from build123d import *

# Parameters (mm, degrees)
SKETCH_1_W          = 26
SKETCH_1_H          = 57.5
SKETCH_1_R          = 1.5
SKETCH_1_R_2        = 6
EXTRUDE_1_DEPTH     = 3
SKETCH_2_W          = 26
SKETCH_2_H          = 3
EXTRUDE_2_DEPTH     = 33
SKETCH_3_W          = 34
SKETCH_3_H          = 60.5
SKETCH_3_R          = 2
SKETCH_3_R_2        = 13
EXTRUDE_3_DEPTH     = 3
FILLET_1_R          = 2
EXTRUDE_4_DEPTH     = 1
FILLET_2_R          = 4
SKETCH_5_R          = 1.5
CUT_EXTRUDE_1_DEPTH = 50.503156465


with BuildPart() as part:
    # 草图1 → 凸台-拉伸1 (new body)
    with BuildSketch(Plane.XY):
        Rectangle(SKETCH_1_W, SKETCH_1_H)
        with Locations((-5, 24.25)):
            Circle(SKETCH_1_R, mode=Mode.SUBTRACT)
        with Locations((5, 24.25)):
            Circle(SKETCH_1_R, mode=Mode.SUBTRACT)
        with Locations((5, -24.25)):
            Circle(SKETCH_1_R, mode=Mode.SUBTRACT)
        with Locations((-5, -24.25)):
            Circle(SKETCH_1_R, mode=Mode.SUBTRACT)
        with Locations((0, 10.25)):
            Circle(SKETCH_1_R_2, mode=Mode.SUBTRACT)
    extrude(amount=EXTRUDE_1_DEPTH)

    # 草图2 → 凸台-拉伸2 (add)
    with BuildSketch(Plane(origin=(0, 0, 0), x_dir=(-1, 0, 0), z_dir=(0, 0, -1))):
        with Locations((0, -30.25)):
            Rectangle(SKETCH_2_W, SKETCH_2_H)
    extrude(amount=-EXTRUDE_2_DEPTH)

    # 草图3 → 凸台-拉伸3 (add)
    with BuildSketch(Plane.XY.offset(33)):
        with Locations((0, -1.5)):
            Rectangle(SKETCH_3_W, SKETCH_3_H)
        with Locations((12.374368671, 22.624368671)):
            Circle(SKETCH_3_R, mode=Mode.SUBTRACT)
        with Locations((12.374368671, -2.124368671)):
            Circle(SKETCH_3_R, mode=Mode.SUBTRACT)
        with Locations((-12.374368671, -2.124368671)):
            Circle(SKETCH_3_R, mode=Mode.SUBTRACT)
        with Locations((-12.374368671, 22.624368671)):
            Circle(SKETCH_3_R, mode=Mode.SUBTRACT)
        with Locations((0, 10.25)):
            Circle(SKETCH_3_R_2, mode=Mode.SUBTRACT)
    extrude(amount=-EXTRUDE_3_DEPTH)

    # 圆角1
    fillet_1_edges = [part.edges().sort_by_distance(p)[0] for p in [
        (0, -28.75, 3),
        (0, -28.75, 30),
    ]]
    fillet(fillet_1_edges, radius=FILLET_1_R)

    # 草图4 → 凸台-拉伸4 (add)
    with BuildSketch(Plane.XZ.offset(31.75)):
        Polygon((13, 0), (13, 30), (17, 30), (17, 33), (-17, 33), (-17, 30), (-13, 30), (-13, 0), align=None)
    extrude(amount=EXTRUDE_4_DEPTH)

    # 圆角2
    fillet_2_edges = [part.edges().sort_by_distance(p)[0] for p in [
        (-13, 28.75, 1.5),
        (13, 28.75, 1.5),
        (-17, 28.75, 31.5),
        (17, 28.75, 31.5),
        (17, -32.75, 31.5),
        (-17, -32.75, 31.5),
    ]]
    fillet(fillet_2_edges, radius=FILLET_2_R)

    # 草图5 → 切除-拉伸1 (cut, through all)
    with BuildSketch(Plane(origin=(0, 0, 0), x_dir=(-1, 0, 0), z_dir=(0, 0, -1))):
        with Locations(Location((-5, -24.25, 0), (0, 0, 180))):
            Circle(SKETCH_5_R)
        with Locations(Location((5, -24.25, 0), (0, 0, 180))):
            Circle(SKETCH_5_R)
        with Locations((-5, -14.244897428)):
            Circle(SKETCH_5_R)
        with Locations((5, -14.244897428)):
            Circle(SKETCH_5_R)
    extrude(amount=-CUT_EXTRUDE_1_DEPTH, mode=Mode.SUBTRACT)


solid = part.part
Part model, mm, in its own coordinate system. A direction names the side the tool comes from. Give positions to 0.01 mm unless a question says otherwise; leave off trailing zeros. Loops run counter-clockwise (first coordinate to the right, second up) from the corner with the lowest first, then second, coordinate; pieces in that order, holes last.
(1) 3-axis set-ups, long thin cutter, end or side, ignore diameter. For faces 1 (the cylindrical face through (-10.316, 2.34, 31.521)), 2 (the cylindrical face through (0.18, -28.15, 3.57)), 3 (the cylindrical face through (-15.859, 27.547, 31.479)): which of +Z, -Z, +X, -X, +Y, -Y reach the whole face in a straight line?
Return value:
face 1: +Z
face 2: +X, -X, +Y
face 3: +Z, -Z, -X, +Y
(2) Pull direction X, two halves, no side cores. Call faces 4 (the flat face through (0, 28.75, 1)), 5 (the cylindrical face through (4.805, -25.737, 31.479)), 6 (the cylindrical face through (11.859, 27.547, 1.521)): pulls with the +X half, pulls with the -X half, needs draft (parallel to the pull), parting line crosses it, or undercut.
Return value:
face 4: needs draft
face 5: undercut
face 6: pulls with the +X half
(3) Band-saw the part on D-D (z = 15.5). Write the cut outline in (x, y), and give its area (3 significant figures).
Return value:
outline: (-13, -32.75) - (13, -32.75) - (13, -28.75) - (-13, -28.75) - close
area: 104 mm2
(4) Band-saw the part on B-B (y = 10.25). Write the cut outline in (x, z).
Return value:
outline: (-17, 30) - (-13, 30) - (-13, 33) - (-17, 33) - close; (-13, 0) - (-6, 0) - (-6, 3) - (-13, 3) - close; (6, 0) - (13, 0) - (13, 3) - (6, 3) - close; (13, 30) - (17, 30) - (17, 33) - (13, 33) - close
(5) Pin check, flat tips, straight feed: pin 1 (3 mm diameter, centred on x = 2, y = 0.5, fed in from +Z); pin 2 (9 mm diameter, centred on y = 2.5, z = 22.5, fed in from -X); pin 3 (7 mm diameter, centred on x = 0.5, z = 15.5, fed in from +Y). Stop position of each tip, or through.
Return value:
pin 1: stops at z = 3
pin 2: passes through
pin 3: stops at y = -28.75
(6) Band-saw the part on A-A (x = 0). Write the cut outline in (y, z), and give its area (3 significant figures).
Return value:
outline: (-32.75, 0) - (4.25, 0) - (4.25, 3) - (-26.75, 3) arc R2 cw to (-28.75, 5) - (-28.75, 28) arc R2 cw to (-26.75, 30) - (-2.75, 30) - (-2.75, 33) - (-32.75, 33) - close; (16.25, 0) - (28.75, 0) - (28.75, 3) - (16.25, 3) - close; (23.25, 30) - (28.75, 30) - (28.75, 33) - (23.25, 33) - close
area: 365 mm2
(7) Drill centre lines: line 1 along Z through (x, y) = (10, 25); line 2 along Y through (x, z) = (5, 2.3); line 3 along Z through (x, y) = (-15, 1). Where is each one in solid material? Low to high.
Return value:
line 1: z = 0 to 3, 30 to 33
line 2: y = -32.75 to -25.75, -22.75 to -15.74, -12.74 to 6.93, 13.57 to 22.75, 25.75 to 28.75
line 3: z = 30 to 33
(8) Band-saw the part on C-C (y = -18). Write the cut outline in (x, z).
Return value:
outline: (-17, 30) - (17, 30) - (17, 33) - (-17, 33) - close; (-13, 0) - (13, 0) - (13, 3) - (-13, 3) - close
